Source: CAD feature listing. Evaluate the final solid. Frame: model axes, mm. A direction names the side the tool comes from. Coordinates: 2 decimals unless noted, no trailing zeros. Order: outer loops, then holes, each group sorted by start corner. A loop starts at its lowest first (then second) coordinate and runs counter-clockwise, first axis right, second up. Notation, with made-up numbers: (65.25, 80) - (93.25, 80) arc R24 cw to (93.25, 93) - close; hole circle Ø7 at (83, 53.5). An arc over 180 degrees is marked (long way). One line per question, with ' | ' between items.
from build123d import *

# Parameters (mm, degrees)
Y_KSEKLIK_EKSTR_ZYON3_DEPTH = 3
KES_EKSTR_ZYON10_DEPTH      = 3
KES_EKSTR_ZYON11_DEPTH      = 3
KES_EKSTR_ZYON14_DEPTH      = 3
KES_EKSTR_ZYON15_DEPTH      = 3
KES_EKSTR_ZYON16_DEPTH      = 3
KES_EKSTR_ZYON17_DEPTH      = 3
KES_EKSTR_ZYON18_DEPTH      = 3
IZIM28_R                    = 1.6
KES_EKSTR_ZYON19_DEPTH      = 3
IZIM29_R                    = 1.6
KES_EKSTR_ZYON20_DEPTH      = 3
IZIM30_R                    = 1.6
KES_EKSTR_ZYON21_DEPTH      = 3
IZIM31_W                    = 41
IZIM31_H                    = 20
KES_EKSTR_ZYON22_DEPTH      = 10
IZIM32_R                    = 1.6
KES_EKSTR_ZYON23_DEPTH      = 10
KES_EKSTR_ZYON24_DEPTH      = 10
IZIM34_R                    = 2.1
KES_EKSTR_ZYON25_DEPTH      = 3
IZIM35_R                    = 1.6
KES_EKSTR_ZYON26_DEPTH      = 45
IZIM36_R                    = 1.6
KES_EKSTR_ZYON27_DEPTH      = 45


with BuildPart() as part:
    # Çizim16 → Yükseklik-Ekstrüzyon3 (new body)
    with BuildSketch(Plane(origin=(0, 0, 0), x_dir=(1, 0, 0), z_dir=(0, 1, 0))):
        with BuildLine():
            Line((-110, -70), (100, -70))
            ThreePointArc((100, -70), (107.071067812, -67.071067812), (110, -60))
            Line((110, -60), (110, 60))
            ThreePointArc((110, 60), (107.071067812, 67.071067812), (100, 70))
            Line((100, 70), (-110, 70))
            Line((-110, 70), (-110, -70))
        make_face()
    extrude(amount=Y_KSEKLIK_EKSTR_ZYON3_DEPTH)

    # Çizim18 → Kes-Ekstrüzyon10 (cut)
    with BuildSketch(Plane(origin=(0, 3, 0), x_dir=(1, 0, 0), z_dir=(0, 1, 0))):
        with BuildLine():
            Line((-19, 70), (-25.463821511, 59.889658192))
            ThreePointArc((-25.463821511, 59.889658192), (-43.144058736, 50.67991016), (-60, 61.323569832))
            ThreePointArc((-60, 61.323569832), (-63.804672609, 66.383043129), (-69, 70))
            Line((-69, 70), (-19, 70))
        make_face()
    extrude(amount=-KES_EKSTR_ZYON10_DEPTH, mode=Mode.SUBTRACT)

    # Çizim19 → Kes-Ekstrüzyon11 (cut)
    with BuildSketch(Plane(origin=(0, 3, 0), x_dir=(1, 0, 0), z_dir=(0, 1, 0))):
        with BuildLine():
            Line((-19, -70), (-25.463821511, -59.889658192))
            ThreePointArc((-25.463821511, -59.889658192), (-43.144058736, -50.67991016), (-60, -61.323569832))
            ThreePointArc((-60, -61.323569832), (-63.804672609, -66.383043129), (-69, -70))
            Line((-69, -70), (-19, -70))
        make_face()
    extrude(amount=-KES_EKSTR_ZYON11_DEPTH, mode=Mode.SUBTRACT)

    # Çizim23 → Kes-Ekstrüzyon14 (cut)
    with BuildSketch(Plane(origin=(0, 3, 0), x_dir=(1, 0, 0), z_dir=(0, 1, 0))):
        with BuildLine():
            Line((-84, -70), (-90.329717397, -53.149638649))
            ThreePointArc((-90.329717397, -53.149638649), (-98.077113424, -40.633105793), (-110, -32))
            Line((-110, -32), (-110, -70))
            Line((-110, -70), (-84, -70))
        make_face()
    extrude(amount=-KES_EKSTR_ZYON14_DEPTH, mode=Mode.SUBTRACT)

    # Çizim24 → Kes-Ekstrüzyon15 (cut)
    with BuildSketch(Plane(origin=(0, 3, 0), x_dir=(1, 0, 0), z_dir=(0, 1, 0))):
        with BuildLine():
            Line((-84, 70), (-90.329717397, 53.149638649))
            ThreePointArc((-90.329717397, 53.149638649), (-98.077113424, 40.633105793), (-110, 32))
            Line((-110, 32), (-110, 70))
            Line((-110, 70), (-84, 70))
        make_face()
    extrude(amount=-KES_EKSTR_ZYON15_DEPTH, mode=Mode.SUBTRACT)

    # Çizim25 → Kes-Ekstrüzyon16 (cut)
    with BuildSketch(Plane(origin=(0, 3, 0), x_dir=(1, 0, 0), z_dir=(0, 1, 0))):
        with BuildLine():
            Line((-44.007256251, -8), (-71.228571429, -30))
            ThreePointArc((-71.228571429, -30), (-75.447541301, -29.552458699), (-75, -25.333488827))
            Line((-75, -25.333488827), (-47.778684822, -3.333488827))
            ThreePointArc((-47.778684822, -3.333488827), (-43.55971495, -3.781030128), (-44.007256251, -8))
        make_face()
    extrude(amount=-KES_EKSTR_ZYON16_DEPTH, mode=Mode.SUBTRACT)

    # Çizim26 → Kes-Ekstrüzyon17 (cut)
    with BuildSketch(Plane(origin=(0, 3, 0), x_dir=(1, 0, 0), z_dir=(0, 1, 0))):
        with BuildLine():
            Line((-71.228571429, 30), (-44.007256251, 8))
            ThreePointArc((-44.007256251, 8), (-43.55971495, 3.781030128), (-47.778684822, 3.333488827))
            Line((-47.778684822, 3.333488827), (-75, 25.333488827))
            ThreePointArc((-75, 25.333488827), (-75.447541301, 29.552458699), (-71.228571429, 30))
        make_face()
    extrude(amount=-KES_EKSTR_ZYON17_DEPTH, mode=Mode.SUBTRACT)

    # Çizim27 → Kes-Ekstrüzyon18 (cut)
    with BuildSketch(Plane(origin=(0, 3, 0), x_dir=(1, 0, 0), z_dir=(0, 1, 0))):
        with BuildLine():
            Line((-15, -3), (-30, -3))
            ThreePointArc((-30, -3), (-33, 0), (-30, 3))
            Line((-30, 3), (-15, 3))
            ThreePointArc((-15, 3), (-12, 0), (-15, -3))
        make_face()
    extrude(amount=-KES_EKSTR_ZYON18_DEPTH, mode=Mode.SUBTRACT)

    # Çizim28 → Kes-Ekstrüzyon19 (cut)
    with BuildSketch(Plane(origin=(0, 3, 0), x_dir=(1, 0, 0), z_dir=(0, 1, 0))):
        with Locations(Location((1, -67, 0), (0, 0, 270))):
            Circle(IZIM28_R)
        with Locations(Location((26.7, -67, 0), (0, 0, 270))):
            Circle(IZIM28_R)
    extrude(amount=-KES_EKSTR_ZYON19_DEPTH, mode=Mode.SUBTRACT)

    # Çizim29 → Kes-Ekstrüzyon20 (cut)
    with BuildSketch(Plane(origin=(0, 3, 0), x_dir=(1, 0, 0), z_dir=(0, 1, 0))):
        with Locations(Location((-107, 12.85, 0), (0, 0, 270))):
            Circle(IZIM29_R)
        with Locations(Location((-107, -12.85, 0), (0, 0, 270))):
            Circle(IZIM29_R)
    extrude(amount=-KES_EKSTR_ZYON20_DEPTH, mode=Mode.SUBTRACT)

    # Çizim30 → Kes-Ekstrüzyon21 (cut)
    with BuildSketch(Plane(origin=(0, 3, 0), x_dir=(1, 0, 0), z_dir=(0, 1, 0))):
        with Locations(Location((1, 67, 0), (0, 0, 270))):
            Circle(IZIM30_R)
        with Locations(Location((26.7, 67, 0), (0, 0, 270))):
            Circle(IZIM30_R)
    extrude(amount=-KES_EKSTR_ZYON21_DEPTH, mode=Mode.SUBTRACT)

    # Çizim31 → Kes-Ekstrüzyon22 (cut)
    with BuildSketch(Plane(origin=(0, 3, 0), x_dir=(1, 0, 0), z_dir=(0, 1, 0))):
        with Locations((-81.5, 0)):
            Rectangle(IZIM31_W, IZIM31_H)
    extrude(amount=-KES_EKSTR_ZYON22_DEPTH, mode=Mode.SUBTRACT)

    # Çizim32 → Kes-Ekstrüzyon23 (cut)
    with BuildSketch(Plane(origin=(0, 3, 0), x_dir=(1, 0, 0), z_dir=(0, 1, 0))):
        with Locations(Location((95, -65, 0), (0, 0, 270))):
            Circle(IZIM32_R)
        with Locations(Location((95, 65, 0), (0, 0, 270))):
            Circle(IZIM32_R)
        with Locations(Location((-95, -28, 0), (0, 0, 270))):
            Circle(IZIM32_R)
        with Locations(Location((-95, 28, 0), (0, 0, 270))):
            Circle(IZIM32_R)
    extrude(amount=-KES_EKSTR_ZYON23_DEPTH, mode=Mode.SUBTRACT)

    # Çizim33 → Kes-Ekstrüzyon24 (cut)
    with BuildSketch(Plane(origin=(0, 3, 0), x_dir=(1, 0, 0), z_dir=(0, 1, 0))):
        with BuildLine():
            Line((97, 46), (-13, 46))
            ThreePointArc((-13, 46), (-19, 52), (-13, 58))
            Line((-13, 58), (97, 58))
            ThreePointArc((97, 58), (103, 52), (97, 46))
        make_face()
        with BuildLine():
            Line((-13, -46), (97, -46))
            ThreePointArc((97, -46), (103, -52), (97, -58))
            Line((97, -58), (-13, -58))
            ThreePointArc((-13, -58), (-19, -52), (-13, -46))
        make_face()
    extrude(amount=-KES_EKSTR_ZYON24_DEPTH, mode=Mode.SUBTRACT)

    # Çizim34 → Kes-Ekstrüzyon25 (cut)
    with BuildSketch(Plane(origin=(0, 3, 0), x_dir=(1, 0, 0), z_dir=(0, 1, 0))):
        with Locations(Location((-75, -60, 0), (0, 0, 270))):
            Circle(IZIM34_R)
        with Locations(Location((-75, 60, 0), (0, 0, 270))):
            Circle(IZIM34_R)
    extrude(amount=-KES_EKSTR_ZYON25_DEPTH, mode=Mode.SUBTRACT)

    # Çizim35 → Kes-Ekstrüzyon26 (cut)
    with BuildSketch(Plane(origin=(0, 3, 0), x_dir=(1, 0, 0), z_dir=(0, 1, 0))):
        with Locations(Location((95, -38, 0), (0, 0, 270))):
            Circle(IZIM35_R)
        with Locations(Location((95, 38, 0), (0, 0, 270))):
            Circle(IZIM35_R)
        with Locations(Location((0, 38, 0), (0, 0, 270))):
            Circle(IZIM35_R)
        with Locations(Location((0, -38, 0), (0, 0, 270))):
            Circle(IZIM35_R)
    extrude(amount=-KES_EKSTR_ZYON26_DEPTH, mode=Mode.SUBTRACT)

    # Çizim36 → Kes-Ekstrüzyon27 (cut)
    with BuildSketch(Plane(origin=(0, 3, 0), x_dir=(1, 0, 0), z_dir=(0, 1, 0))):
        with Locations(Location((0, 25, 0), (0, 0, 270))):
            Circle(IZIM36_R)
        with Locations(Location((58, 25, 0), (0, 0, 270))):
            Circle(IZIM36_R)
        with Locations(Location((0, -24, 0), (0, 0, 270))):
            Circle(IZIM36_R)
        with Locations(Location((58, -24, 0), (0, 0, 270))):
            Circle(IZIM36_R)
    extrude(amount=-KES_EKSTR_ZYON27_DEPTH, mode=Mode.SUBTRACT)


solid = part.part
(1) Set-up query: faces 4 (the flat face through (-22.187, 1.521, -65.016)), 5 (the flat face through (-22.187, 1.521, 65.016)), 6 (the flat face through (-57.808, 1.521, -19.154)). Return all of +Z, -Z, +X, -X, +Y, -Y with unobstructed straight access to the full face (end or side cutting, diameter ignored); none if empty.
Taken from the geometry:
face 4: -Z, +Y, -Y | face 5: +Z, +Y, -Y | face 6: +Y, -Y
(2) Cut plane D-D (y = 2.5). State how many separate pieces and enclosed holes the cut face has, and give its area (3 significant figures).
Taken from the geometry:
separate pieces: 1 | enclosed holes: 26 | area: 23,700 mm²
(3) Cut plane A-A (x = 34.5). Return the cut outline in (y, z).
Taken from the geometry:
outline: (0, -70) - (3, -70) - (3, -58) - (0, -58) - close; (0, -46) - (3, -46) - (3, 46) - (0, 46) - close; (0, 58) - (3, 58) - (3, 70) - (0, 70) - close
(4) Cut plane B-B (z = -20). Return the cut outline in (x, y), and give its area (3 significant figures).
Taken from the geometry:
outline: (-110, 0) - (-68.4, 0) - (-68.4, 3) - (-110, 3) - close; (-58.86, 0) - (110, 0) - (110, 3) - (-58.86, 3) - close | area: 631 mm²
(5) Pull-direction query (X, two-part tool) for faces 1 (the cylindrical face through (107.15, 1.48, -66.99)), 2 (the cylindrical face through (-97.936, 1.521, -40.785)), 3 (the flat face through (-61.58, 1.52, 14.49)); classes: pulls with the +X half, pulls with the -X half, needs draft (parallel to the pull), parting line crosses it, or undercut.
Taken from the geometry:
face 1: pulls with the +X half | face 2: pulls with the -X half | face 3: undercut
(6) Material intervals for L1, parallel to Z at x = 24, y = 1.25; L2, parallel to X at y = 1.1, z = 60 (3 decimals); L3, parallel to X at y = 1.75, z = -54.5, sorted ascending. Write a range as from..to.
Taken from the geometry:
L1: z = -70..-58, -46..46, 58..70 | L2: x = -87.756..-77.1, -72.9..-59.235, -25.393..110 | L3: x = -89.82..-54.09, -30.53..-18.45, 102.45..110
(7) Cut plane C-C (x = -66). Return the cut outline in (y, z).
Taken from the geometry:
outline: (0, -68.22) - (3, -68.22) - (3, -25.77) - (0, -25.77) - close; (0, -18.06) - (3, -18.06) - (3, -10) - (0, -10) - close; (0, 10) - (3, 10) - (3, 18.06) - (0, 18.06) - close; (0, 25.77) - (3, 25.77) - (3, 68.22) - (0, 68.22) - close
